Autodesk Inventor part; units mm, degrees
ref_plane "YZ Plane" through (0, 0, 0) normal (1, 0, 0) x (0, 1, 0)
ref_plane "XZ Plane" through (0, 0, 0) normal (0, 1, 0) x (-1, 0, 0)
ref_plane "XY Plane" through (0, 0, 0) normal (0, 0, 1) x (1, 0, 0)
sketch "Sketch12" plane through (0, 0, 0) normal (0, 0, -1) x (-1, 0, 0)
  line L0 (0, 0) -> (-80, 0)
  line L1 (-80, 0) -> (-80, -120)
  line L2 (-80, -120) -> (0, -120)
  line L3 (0, -120) -> (0, 0)
  line L4 (-80, 0) -> (-36.3011, 0)
  line L5 (-36.3011, 0) -> (-36.3011, -79.996)
  line L6 (-36.3011, -79.996) -> (-80, -79.996)
  line L7 (-80, -79.996) -> (-80, 0)
  point P0 (-36.3011, 0)
  point P1 (-80, -79.996)
  dimension "d107" = 80
  dimension "d108" = 120
sketch "Sketch1" plane through (0, 0, 0) normal (0, 0, 1) x (1, 0, 0)
  line L0 (0, 0) -> (-350, 0)
  line L1 (0, -80) -> (0, 0)
  line L2 (-350, 0) -> (-350, -80)
  line L3 (-350, -80) -> (0, -80)
  point P0 (0, -40)
  dimension "d32" = 80
  dimension "d60" = 80
  dimension "d61" = 350
extrude "Plate1" add sketch "Sketch1" along normal blind 2
sketch "Sketch11" plane through (0, 0, 0) normal (0, 0, -1) x (-1, 0, 0)
  line L0 (60.25, -48.25) -> (29.75, -48.25)
  line L1 (29.75, -48.25) -> (29.75, -17.75)
  line L2 (29.75, -17.75) -> (60.25, -17.75)
  line L3 (60.25, -17.75) -> (60.25, -48.25)
  line L4 (60.25, -48.25) -> (29.75, -17.75) construction
  line L5 (29.75, -48.25) -> (60.25, -17.75) construction
  circle A0 centre (68, -56) radius 2.5
  circle A1 centre (22, -56) radius 2.5
  circle A2 centre (22, -10) radius 2.5
  circle A3 centre (68, -10) radius 2.5
  line L6 (29.75, -48.25) -> (22, -56) construction
  line L7 (0, -80) -> (0, 0)
  line L8 (0, 0) -> (350, 0)
  line L9 (350, -80) -> (0, -80)
  line L10 (22, -10) -> (68, -10) construction
  line L11 (68, -10) -> (68, -56) construction
  line L12 (68, -56) -> (22, -56) construction
  line L13 (22, -56) -> (22, -10) construction
  point P0 (45, -33)
  dimension "d88" = 30.5
  dimension "d89" = 30.5
  dimension "d90" = 5
  dimension "d92" = 10.9602
  dimension "d95" = 45
  dimension "d105" = 46
  dimension "d106" = 10
extrude "Extrusion2" cut sketch "Sketch11" against normal through all
sketch "Sketch9" plane through (-350, -78, 0) normal (0, -1, 0) x (1, 0, 0)
  line L0 (350, 0) -> (0, 0)
  line L1 (0, 0) -> (0, -64)
  line L2 (0, -64) -> (350, -64)
  line L3 (350, -64) -> (350, 0)
edge flange "Flange3" height 64 angle 90 thickness 2 bend radius 2.75 thickness toward (0, -1, 0) relief round relief width 2 relief depth 1 edges at (-175, -80, 0) wall of the first edge with corners at (0, -78, 0) (-350, -78, 0) (-350, -78, 64) (0, -78, 64)
bend "Bend3"
corner "Corner3"
pattern_linear "Rectangular Pattern2" count 3 spacing 120 along (-1, 0, 0) of "Extrusion2"
sheet face with bend "Face3" sketch "Sketch12" thickness 2 toward (0, 0, 1) bend radius 2.75 contours L3 L2 L1 L6 L5 L0
bend "Bend5"
equation "\"d2\" = Thickness"
equation "\"d62\" = BendReliefWidth"
equation "\"d63\" = BendReliefDepth"
equation "\"d64\" = MinimumRemnant"
equation "\"d65\" = TransitionRadius"
equation "\"d66\" = MAIN_7_central_window_width + 2 * Thickness"
equation "\"d68\" = BendRadius"
equation "\"d69\" = CornerReliefSize"
equation "\"d70\" = GapSize"
equation "\"d71\" = JacobiRadiusSize"
equation "\"BendReliefWidth\" = Thickness"
equation "\"BendReliefDepth\" = 0.5 * Thickness"
equation "\"CornerReliefSize\" = 4 * Thickness"
equation "\"MinimumRemnant\" = 2 * Thickness"
equation "\"TransitionRadius\" = BendRadius"
equation "\"JacobiRadiusSize\" = BendRadius"
equation "\"GapSize\" = Thickness"
properties part number "PRS-1423 BOTTOM FDS diameter way down_CPY" material "Stainless Steel"
Check sheet for the modelled part. Datum: model origin and axes. Units: mm. A direction names the side the tool comes from. Round coordinates to 2 decimals unless told otherwise and drop trailing zeros. Order: outer loops, then holes, each group sorted by start corner. A loop starts at its lowest first (then second) coordinate and runs counter-clockwise, first axis right, second up.
1) Section check C-C (z = 54.5). Record the boundary of the cut face in (x, y), and give its area (3 significant figures).
2) Go/stop test with flat-tipped pins: pin 1 Ø1.6 at (x, z) = (-158, 1) entering from -Y; pin 2 Ø6 at (x, y) = (-291, -74.5) entering from +Z; pin 3 Ø6 at (x, y) = (-68, -56) entering from +Z; pin 4 Ø4.5 at (x, y) = (-308, -56) entering from -Z. Record where each tip stops, or that it passes through.
3) Section check A-A (y = -38.5). Record the boundary of the cut face in (x, z).
4) Section check B-B (x = -161). Record the boundary of the cut face in (y, z), and give its area (3 significant figures).
5) Scan lines: line 1 (Y direction, x = -142, z = 0.75); line 2 (Y direction, x = -142, z = 0.95); line 3 (Y direction, x = -237, z = 43). Record each from-to range of solid material in increasing order.
6) Tool access check on faces 1 (the flat face through (-350, -58, 1)), 2 (the flat face through (-173, -78, 34)). Record the directions out of +Z, -Z, +X, -X, +Y, -Y that give a thin tool (end or side, any length) a straight path to the whole face; none if there is none.
Result:
1. outline: (-350, -80) - (0, -80) - (0, -78) - (-350, -78) - close
1. area: 700 mm2
2. pin 1: stops at y = -78.97
2. pin 2: stops at z = 3.17
2. pin 3: stops at z = 2
2. pin 4: passes through
3. outline: (-350, 0) - (-300.25, 0) - (-300.25, 2) - (-350, 2) - close; (-269.75, 0) - (-180.25, 0) - (-180.25, 2) - (-269.75, 2) - close; (-149.75, 0) - (-60.25, 0) - (-60.25, 2) - (-149.75, 2) - close; (-29.75, 0) - (36.3, 0) - (36.3, 2) - (-29.75, 2) - close
4. outline: (-80, 4.75) arc R4.75 ccw to (-75.25, 0) - (-48.25, 0) - (-48.25, 2) - (-75.25, 2) arc R2.75 cw to (-78, 4.75) - (-78, 64) - (-80, 64) - close; (-17.75, 0) - (0, 0) - (0, 2) - (-17.75, 2) - close
4. area: 220 mm2
5. line 1: y = -77.81 to -58.5, -53.5 to -12.5, -7.5 to 0
5. line 2: y = -78.1 to -58.5, -53.5 to -12.5, -7.5 to 0
5. line 3: y = -80 to -78
6. face 1: +Z, -Z, -X, +Y, -Y
6. face 2: +Z, +X, -X, +Y
